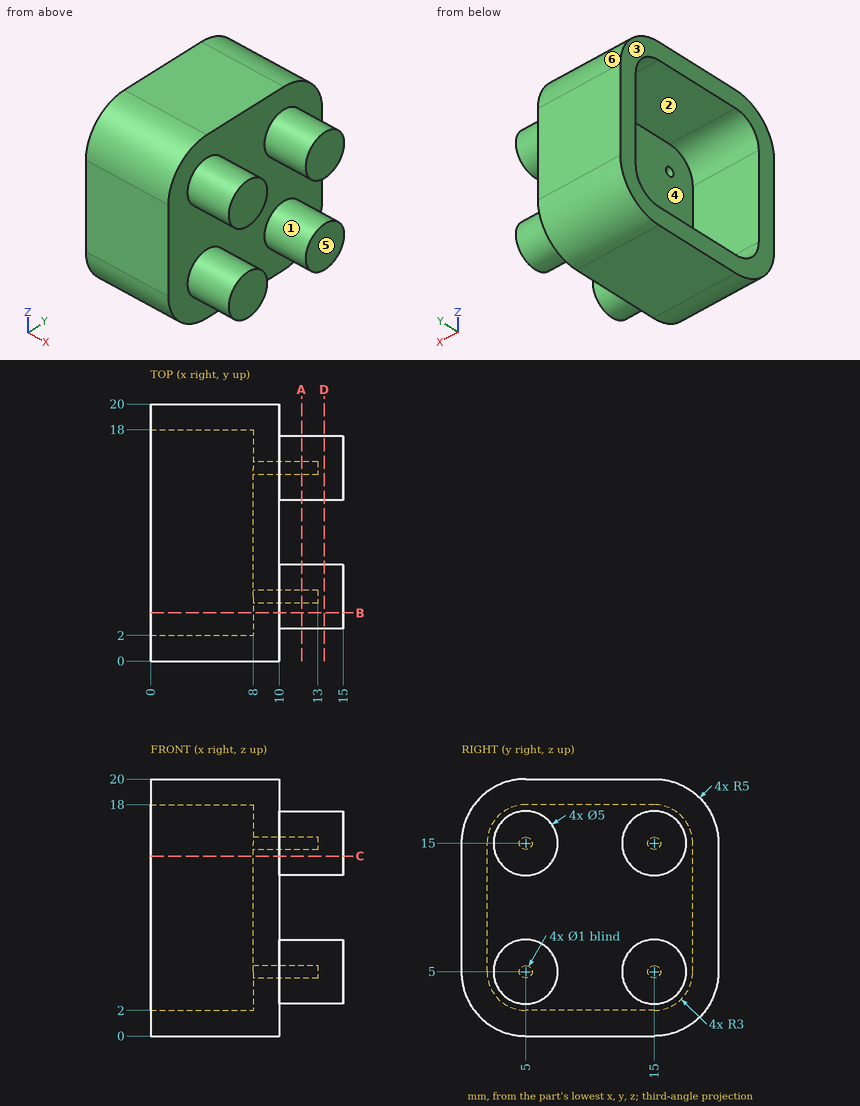
Geometry: see drawing. Coordinates: mm, zero at the bounding-box minimum. A direction names the side the tool comes from. Give positions to 0.01 mm unless a question says otherwise; leave off trailing zeros. Loops run counter-clockwise (first coordinate to the right, second up) from the corner with the lowest first, then second, coordinate; pieces in that order, holes last. Notation, with made-up numbers: (-34.75, 12.25) - (-29.75, 12.25) arc R29 cw to (-29.75, 35.25) - close; hole circle Ø11 at (-33, -15.5). An arc over 180 degrees is marked (long way). Answer as CSV lines item,"result". Start each with the question number.
1. Section D-D, the plane x = 13.5. Return loops of the section in (y, z).
2. Pin query (flat end, axial travel): P1, Ø4, axis at x = 6.5, y = 16.5, coming from the -Z side; P2, Ø1, axis at y = 9.5, z = 11, coming from the +X side; P3, Ø1.1, axis at y = 15, z = 5, coming from the -X side; P4, Ø0.5, axis at y = 5, z = 15, coming from the -X side. Return the tip coordinate at first contact, or that it passes through.
3. Section A-A, the plane x = 11.75. Return loops of the section in (y, z), plus the area to 3 significant figures.
4. Ray query, L1, parallel to Y at x = 9.8, z = 5; L2, parallel to Y at x = 1, z = 14; L3, parallel to X at y = 13, z = 11.5. Return the intervals inside material, ascending.
5. Reachability of the marked faces 1, 2 and 3 from +Z, -Z, +X, -X, +Y, -Y: full face, straight path, thin tool, end or side. Return the list, or none.
6. Section C-C, the plane z = 14. Return loops of the section in (x, y).
7. Draft query along Y for the marked faces 4, 5 and 6. Return one class per face: released by +Y, released by -Y, zero draft, split by the parting line, or undercut.
8. Section B-B, the plane y = 3.75. Return loops of the section in (x, z), plus the area to 3 significant figures.
Answers:
1,outline,"circle Ø5 at (5, 5); circle Ø5 at (5, 15); circle Ø5 at (15, 5); circle Ø5 at (15, 15)"
2,P1,"stops at z = 0"
2,P2,"stops at x = 10"
2,P3,"stops at x = 8"
2,P4,"stops at x = 13"
3,outline,"circle Ø5 at (5, 5); circle Ø5 at (5, 15); circle Ø5 at (15, 5); circle Ø5 at (15, 15); hole circle Ø1 at (5, 5); hole circle Ø1 at (5, 15); hole circle Ø1 at (15, 5); hole circle Ø1 at (15, 15)"
3,area,"75.4 mm2"
4,L1,"y = 0 to 4.5, 5.5 to 14.5, 15.5 to 20"
4,L2,"y = 0 to 2, 18 to 20"
4,L3,"x = 8 to 10"
5,face 1,"+X"
5,face 2,"-X"
5,face 3,"+Z, -Z, -X, +Y, -Y"
6,outline,"(0, 0) - (10, 0) - (10, 2.71) - (15, 2.71) - (15, 7.29) - (10, 7.29) - (10, 12.71) - (15, 12.71) - (15, 17.29) - (10, 17.29) - (10, 20) - (0, 20) - (0, 18) - (8, 18) - (8, 2) - (0, 2) - close"
7,face 4,"undercut"
7,face 5,"zero draft"
7,face 6,"released by +Y"
8,outline,"(0, 0.16) - (10, 0.16) - (10, 2.83) - (15, 2.83) - (15, 7.17) - (10, 7.17) - (10, 12.83) - (15, 12.83) - (15, 17.17) - (10, 17.17) - (10, 19.84) - (0, 19.84) - (0, 17.73) - (8, 17.73) - (8, 2.27) - (0, 2.27) - close"
8,area,"116 mm2"
